```python
from build123d import *

# Parameters (mm, degrees)
SKETCH1_R           = 55
BOSS_EXTRUDE1_DEPTH = 48
SKETCH2_R           = 50
CUT_EXTRUDE1_DEPTH  = 49
SKETCH5_W           = 106
SKETCH5_H           = 5.5
CUT_EXTRUDE2_DEPTH  = 45


with BuildPart() as part:
    # Sketch1 → Boss-Extrude1 (new body)
    with BuildSketch(Plane.XY):
        Circle(SKETCH1_R)
    extrude(amount=BOSS_EXTRUDE1_DEPTH)

    # Sketch2 → Cut-Extrude1 (cut, through all)
    with BuildSketch(Plane.XY.offset(48)):
        Circle(SKETCH2_R)
    extrude(amount=-CUT_EXTRUDE1_DEPTH, mode=Mode.SUBTRACT)

    # Sketch5 → Cut-Extrude2 (cut)
    with BuildSketch(Plane.XY.offset(48)):
        with Locations((0, -7.75)):
            Rectangle(SKETCH5_W, SKETCH5_H)
    extrude(amount=-CUT_EXTRUDE2_DEPTH, mode=Mode.SUBTRACT)


solid = part.part
```
Part model, mm, in its own coordinate system. A direction names the side the tool comes from. Coordinates: 2 decimals unless noted, no trailing zeros. Order: outer loops, then holes, each group sorted by start corner. A loop starts at its lowest first (then second) coordinate and runs counter-clockwise, first axis right, second up. Notation, with made-up numbers: (31.25, -20) -> (48.25, -20) arc R7 ccw to (48.25, -9) -> close; hole circle Ø10 at (78, 40.25). An arc over 180 degrees is marked (long way). Put each result on its own line as item: value. Start each with the question number.
(1) Pin check, flat tips, straight feed: pin 1 Ø4.5 at (x, z) = (50.5, 30) entering from +Y; pin 2 Ø1.6 at (y, z) = (-8.5, 17) entering from -X; pin 3 Ø1.6 at (x, z) = (51.5, 34) entering from -Y. Stop position of each tip, or through.
(2) Band-saw the part on A-A (z = 17). Give the cut face in (x, y), then the cut area to 3 significant figures.
(3) Mould opens along Y. For faces 3 (the face through (12, -49, 0)), 4 (the face through (-11.923, -53.692, 23.664)), 5 (the face through (53, -8, 26)) say: pulls with the +Y half, pulls with the -Y half, needs draft (parallel to the pull), parting line crosses it, or undercut.
(4) Band-saw the part on B-B (y = 0). Give the cut face in (x, z), then the cut area to 3 significant figures.
(5) Probe line 1 along Y through (x, z) = (0, 29); line 2 along X through (y, z) = (39, 43.5); line 3 along X through (y, z) = (-12.5, 2). List the from-to ranges inside material, lowest first. Write a range as [from, to].
(6) Which spindle directions (+Z, -Z, +X, -X, +Y, -Y) get a long thin tool onto all of the face, cutting with end or side? Do faces 1 (the face through (47.69, 15.02, 24.34)), 2 (the face through (-51, -10.5, 26)). Say none if no direction does.
Determined:
1. pin 1: stops at y = 26.4
1. pin 2: stops at x = -54.46
1. pin 3: stops at y = -21.32
2. outline: circle Ø110 at (0, 0); hole (-53, -10.5) -> (-48.89, -10.5) arc R50 ccw to (48.89, -10.5) -> (53, -10.5) -> (53, -5) -> (49.75, -5) arc R50 ccw (long way) to (-49.75, -5) -> (-53, -5) -> close
2. area: 1,610 mm²
3. face 3: needs draft
3. face 4: parting line crosses it
3. face 5: undercut
4. outline: (-55, 0) -> (-50, 0) -> (-50, 48) -> (-55, 48) -> close; (50, 0) -> (55, 0) -> (55, 48) -> (50, 48) -> close
4. area: 480 mm²
5. line 1: y = [-55, -50], [50, 55]
5. line 2: x = [-38.78, -31.29], [31.29, 38.78]
5. line 3: x = [-53.56, -48.41], [48.41, 53.56]
6. face 1: +Z, -Z
6. face 2: +Z
